Geometry check sheet. Reference: the model listing, model coordinates, mm. A direction names the side the tool comes from. Give positions to 0.01 mm unless a question says otherwise; leave off trailing zeros. Loops run counter-clockwise (first coordinate to the right, second up) from the corner with the lowest first, then second, coordinate; pieces in that order, holes last. Notation, with made-up numbers: (6.25, 51.25) - (50.25, 51.25) arc R9 ccw to (50.25, 66.25) - close; hole circle Ø11 at (0.5, -28.75). An arc over 180 degrees is marked (long way). Use a Markdown table: item, result. Add a question column.
1. Cross-section at B-B on y = -25.4. Count the separate pieces of the cut face and the enclosed holes in it, and give its area (3 significant figures).
2. Set-up check for faces 1 (the flat face through (34, -27.305, 3)), 2 (the cylindrical face through (7.704, -24.063, 2.661)), 3 (the flat face through (-60, -37.338, 3)): record each of +Z, -Z, +X, -X, +Y, -Y from which the full face is reachable in a straight line by a thin tool's end or side.
3. Draft check along Y on faces 4 (the cylindrical face through (0.41, -22.25, 2.74)), 5 (the cylindrical face through (9.5, -20.7, 2.7)), 6 (the flat face through (27.88, -24, 3)). Enter one of: pulls with the +Y half, pulls with the -Y half, needs draft (parallel to the pull), parting line crosses it, or undercut.
4. Cross-section at D-D on x = -15. Enter the section's corners in (y, z), and give its area (3 significant figures).
5. Material ranges on L1, parallel to Y at x = -47, z = 0.8 (3 decimals); L2, parallel to Y at x = 24.5, z = 1.3 (3 decimals); L3, parallel to X at y = -33, z = 2.6, recorded low to high.
6. Cross-section at C-C on x = 46.99. Enter the section's corners in (y, z) (1 decimal), and give its area (3 significant figures).
7. Cross-section at A-A on y = -40. Enter the section's corners in (x, z), and give its area (3 significant figures).
8. Depth check by flat-ended pin: P1, Ø3, axis at y = -24.5, z = 1.5, coming from the -X side; P2, Ø1.6, axis at y = -23.5, z = 2.5, coming from the +X side; P3, Ø8.5, axis at x = 46.99, y = -25.4, coming from the +Z side; P4, Ø1.6, axis at x = -61.5, z = 3, coming from the +Y side. Enter the tip coordinate at first touch or a pass-through.
from build123d import *

# Parameters (mm, degrees)
SKETCH1_R                 = 1.651
BOSS_EXTRUDE2_DEPTH       = 5.3975
SKETCH2_R                 = 1.143
CUT_EXTRUDE1_DEPTH        = 6.3975
SKETCH3_R                 = 12.1285
CUT_EXTRUDE2_DEPTH        = 6.3975
SKETCH4_W                 = 28.562713242
SKETCH4_H                 = 11.677503754
BOSS_EXTRUDE3_DEPTH       = 5.3975
SKETCH5_W                 = 216.7214489
SKETCH5_H                 = 130.569220634
CUT_EXTRUDE4_DEPTH        = 6.3975
SKETCH6_R                 = 38.1
CUT_EXTRUDE5_DEPTH        = 60.96
FILLET1_R                 = 6.35
FILLET2_R                 = 6.35
SKETCH102_W               = 11.43
SKETCH102_H               = 10.16
CUT_EXTRUDE101_DEPTH      = 6.3975001
SKETCH158_R               = 1.651
CUT_EXTRUDE157_DEPTH      = 97.79
SKETCH212_R               = 3.175
CUT_EXTRUDE211_DEPTH      = 103.378
CUT_EXTRUDE211_DEPTH_BACK = 48.768
CUT_EXTRUDE104_DEPTH      = 10
FILLET3_R                 = 2.54


with BuildPart() as part:
    # Sketch1 → Boss-Extrude2 (new body)
    with BuildSketch(Plane.XY):
        with BuildLine():
            Line((-64.964441474, 37.338), (-54.550441474, 37.338))
            Line((-54.550441474, 37.338), (-54.550441474, -37.338))
            Line((-54.550441474, -37.338), (-64.964441474, -37.338))
            ThreePointArc((-64.964441474, -37.338), (0, -74.93), (64.964441474, -37.338))
            Line((64.964441474, -37.338), (54.550441474, -37.338))
            Line((54.550441474, -37.338), (54.550441474, 37.338))
            Line((54.550441474, 37.338), (64.964441474, 37.338))
            ThreePointArc((64.964441474, 37.338), (0, 74.93), (-64.964441474, 37.338))
        make_face()
        with Locations((-46.482, 11.049)):
            Circle(SKETCH1_R, mode=Mode.SUBTRACT)
        with Locations((-21.083270032, 10.795)):
            Circle(SKETCH1_R, mode=Mode.SUBTRACT)
        with Locations((-21.083270032, -10.795)):
            Circle(SKETCH1_R, mode=Mode.SUBTRACT)
        with Locations((-46.482, -11.049)):
            Circle(SKETCH1_R, mode=Mode.SUBTRACT)
        with Locations((46.482, -11.049)):
            Circle(SKETCH1_R, mode=Mode.SUBTRACT)
        with Locations((21.083270032, -10.795)):
            Circle(SKETCH1_R, mode=Mode.SUBTRACT)
        with Locations((21.083270032, 10.795)):
            Circle(SKETCH1_R, mode=Mode.SUBTRACT)
        with Locations((46.482, 11.049)):
            Circle(SKETCH1_R, mode=Mode.SUBTRACT)
    extrude(amount=BOSS_EXTRUDE2_DEPTH)

    # Sketch2 → Cut-Extrude1 (cut, through all)
    with BuildSketch(Plane.XY.offset(5.3975)):
        with Locations((-6.731, 62.23)):
            Circle(SKETCH2_R)
        with Locations((6.731, 62.23)):
            Circle(SKETCH2_R)
    extrude(amount=-CUT_EXTRUDE1_DEPTH, mode=Mode.SUBTRACT)

    # Sketch3 → Cut-Extrude2 (cut, through all)
    with BuildSketch(Plane(origin=(0, 0, 0), x_dir=(-1, 0, 0), z_dir=(0, 0, -1))):
        with Locations((-43.105229381, -43.105229381)):
            Circle(SKETCH3_R)
        with Locations((14.224, -34.29)):
            Circle(SKETCH3_R)
        with Locations((14.224, 34.29)):
            Circle(SKETCH3_R)
        with Locations((-43.105229381, 43.105229381)):
            Circle(SKETCH3_R)
        with Locations((43.105229381, 43.105229381)):
            Circle(SKETCH3_R)
        with Locations((-14.224, 34.29)):
            Circle(SKETCH3_R)
        with Locations((-14.224, -34.29)):
            Circle(SKETCH3_R)
        with Locations((43.105229381, -43.105229381)):
            Circle(SKETCH3_R)
    extrude(amount=-CUT_EXTRUDE2_DEPTH, mode=Mode.SUBTRACT)

    # Sketch4 → Boss-Extrude3 (add)
    with BuildSketch(Plane(origin=(0, 0, 0), x_dir=(-1, 0, 0), z_dir=(0, 0, -1))):
        with Locations((-1.488809975, 62.152540216)):
            Rectangle(SKETCH4_W, SKETCH4_H)
    extrude(amount=-BOSS_EXTRUDE3_DEPTH)

    # Sketch5 → Cut-Extrude4 (cut, through all)
    with BuildSketch(Plane(origin=(0, 0, 0), x_dir=(-1, 0, 0), z_dir=(0, 0, -1))):
        with Locations((23.316688373, 48.139610317)):
            Rectangle(SKETCH5_W, SKETCH5_H)
    extrude(amount=-CUT_EXTRUDE4_DEPTH, mode=Mode.SUBTRACT)

    # Sketch6 → Cut-Extrude5 (cut)
    with BuildSketch(Plane(origin=(0, 0, 0), x_dir=(-1, 0, 0), z_dir=(0, 0, -1))):
        with Locations((0, -86.312058398)):
            Circle(SKETCH6_R)
    extrude(amount=-CUT_EXTRUDE5_DEPTH, mode=Mode.SUBTRACT)

    # Fillet1
    fillet1_edges = [part.edges().sort_by_distance(p)[0] for p in [
        (-33.000960548, -67.271401821, 2.69875),
    ]]
    fillet(fillet1_edges, radius=FILLET1_R)

    # Fillet2
    fillet2_edges = [part.edges().sort_by_distance(p)[0] for p in [
        (33.000960548, -67.271401821, 2.69875),
    ]]
    fillet(fillet2_edges, radius=FILLET2_R)

    # Sketch102 → Cut-Extrude101 (cut, through all)
    with BuildSketch(Plane(origin=(0, 0, 0), x_dir=(-1, 0, 0), z_dir=(0, 0, -1))):
        with Locations((-33.595441474, -22.225)):
            Rectangle(SKETCH102_W, SKETCH102_H)
        with Locations((33.595441474, -22.225)):
            Rectangle(SKETCH102_W, SKETCH102_H)
    extrude(amount=-CUT_EXTRUDE101_DEPTH, mode=Mode.SUBTRACT)

    # Sketch158 → Cut-Extrude157 (cut)
    with BuildSketch(Plane(origin=(30.092005081, 4.08352975, -24.638), x_dir=(-1, 0, 0), z_dir=(0, 0, -1))):
        with Locations((4.154396091, -49.728759131)):
            Circle(SKETCH158_R)
        with Locations((56.02961407, -49.728759131)):
            Circle(SKETCH158_R)
    extrude(amount=-CUT_EXTRUDE157_DEPTH, mode=Mode.SUBTRACT)

    # Sketch212 → Cut-Extrude211 (cut, two sides)
    with BuildSketch(Plane(origin=(30.092005081, 4.08352975, 11.4935), x_dir=(-1, 0, 0), z_dir=(0, 0, -1))) as cut_extrude211_sk:
        with Locations((77.082005081, -29.48352975)):
            Circle(SKETCH212_R)
        with Locations((30.092005081, -29.48352975)):
            Circle(SKETCH212_R)
        with Locations((-16.897994919, -29.48352975)):
            Circle(SKETCH212_R)
    extrude(amount=CUT_EXTRUDE211_DEPTH, mode=Mode.SUBTRACT)
    extrude(cut_extrude211_sk.sketch, amount=-CUT_EXTRUDE211_DEPTH_BACK, mode=Mode.SUBTRACT)

    # Sketch105 → Cut-Extrude104 (cut)
    with BuildSketch(Plane(origin=(0, 0, 0), x_dir=(-1, 0, 0), z_dir=(0, 0, -1))):
        with BuildLine():
            Line((-12.7, -20.32), (-8.89, -20.32))
            ThreePointArc((-8.89, -20.32), (-5.715, -23.495), (-2.54, -20.32))
            Line((-2.54, -20.32), (2.54, -20.32))
            ThreePointArc((2.54, -20.32), (5.715, -23.495), (8.89, -20.32))
            Line((8.89, -20.32), (12.7, -20.32))
            ThreePointArc((12.7, -20.32), (18.415, -14.605), (12.7, -8.89))
            Line((12.7, -8.89), (-12.7, -8.89))
            ThreePointArc((-12.7, -8.89), (-18.415, -14.605), (-12.7, -20.32))
        make_face()
    extrude(amount=-CUT_EXTRUDE104_DEPTH, mode=Mode.SUBTRACT)

    # Fillet3
    fillet3_edges = [part.edges().sort_by_distance(p)[0] for p in [
        (39.310441474, -17.145, 2.69875),
        (27.880441474, -17.145, 2.69875),
        (-27.880441474, -17.145, 2.69875),
        (-39.310441474, -17.145, 2.69875),
        (17.81953367, -17.145, 2.69875),
        (-17.81953367, -17.145, 2.69875),
        (-8.89, -20.32, 2.69875),
        (-2.54, -20.32, 2.69875),
        (2.54, -20.32, 2.69875),
        (8.89, -20.32, 2.69875),
    ]]
    fillet(fillet3_edges, radius=FILLET3_R)


solid = part.part
Values found:
| question | item | result |
|---|---|---|
| 1 | separate pieces | 8 |
| 1 | enclosed holes | 0 |
| 1 | area | 185 mm2 |
| 2 | face 1 | +Z, -Z, +Y |
| 2 | face 2 | +Z, -Z |
| 2 | face 3 | +Z, -Z, -X, +Y |
| 3 | face 4 | undercut |
| 3 | face 5 | pulls with the +Y half |
| 3 | face 6 | needs draft |
| 4 | outline | (-51.29, 0) - (-46.39, 0) - (-46.39, 5.4) - (-51.29, 5.4) - close; (-22.19, 0) - (-19.84, 0) - (-19.84, 5.4) - (-22.19, 5.4) - close |
| 4 | area | 39.1 mm2 |
| 5 | L1 | y = -58.357 to -54.591, -31.619 to -28.575, -22.225 to -17.145 |
| 5 | L2 | y = -57.134 to -46.457, -44.833 to -40.732, -27.848 to -17.145 |
| 5 | L3 | x = -54.55 to -49.81, -36.4 to -26.28, -2.16 to 2.16, 26.28 to 36.4, 49.81 to 54.55 |
| 6 | outline | (-58.4, 0) - (-54.6, 0) - (-54.6, 5.4) - (-58.4, 5.4) - close; (-31.6, 0) - (-28.6, 0) - (-28.6, 5.4) - (-31.6, 5.4) - close; (-22.2, 0) - (-17.1, 0) - (-17.1, 5.4) - (-22.2, 5.4) - close |
| 6 | area | 64.2 mm2 |
| 7 | outline | (-63.36, 0) - (-54.83, 0) - (-54.83, 5.4) - (-63.36, 5.4) - close; (-31.38, 0) - (-24.92, 0) - (-24.92, 5.4) - (-31.38, 5.4) - close; (-3.52, 0) - (3.52, 0) - (3.52, 5.4) - (-3.52, 5.4) - close; (24.92, 0) - (31.38, 0) - (31.38, 5.4) - (24.92, 5.4) - close; (54.83, 0) - (63.36, 0) - (63.36, 5.4) - (54.83, 5.4) - close |
| 7 | area | 200 mm2 |
| 8 | P1 | stops at x = -54.55 |
| 8 | P2 | stops at x = 54.55 |
| 8 | P3 | stops at z = 5.4 |
| 8 | P4 | stops at y = -37.34 |
